Can you work these out from the model? Positions are in its coordinate system, mm. A direction names the side the tool comes from. Give positions to 0.01 mm unless a question says otherwise; leave off trailing zeros. Loops run counter-clockwise (first coordinate to the right, second up) from the corner with the lowest first, then second, coordinate; pieces in that order, holes last. Notation, with made-up numbers: M 66.5,1.25 L 122.5,1.25 A15 cw 122.5,29.25 Z; hole C -20.75,56 d5. An arc over 180 degrees is marked long. Put each result on its own line as item: value. Start each with the question number.
1) Imagine slicing it at B-B (z = -87.5). Write out the boundary of the cut face in (x, y).
2) For faces 1 (the cylindrical face through (2.535, 85.09, 84.615)), 2 (the flat face through (3, 0, -85)), which set-ups out of +Z, -Z, +X, -X, +Y, -Y let a thin tool reach every point of the face, with its end or its side?
3) If we mould it in two halves opening along Y, with no side actions, what happens to faces 3 (the flat face through (3, 10, 0)), 4 (the flat face through (2, 100, 1)), 5 (the flat face through (0, 1, 1))? For each: +Y half, -Y half, draft (parallel to the pull), parting line (faces both ways), or undercut.
4) Imagine slicing it at D-D (x = 1.5). State how many separate pieces and enclosed holes the cut face has, then the cut area to 3 significant figures.
5) Imagine slicing it at C-C (y = 74). Write out the boundary of the cut face in (x, z).
6) Please list where these lines run through material, in increasing order: line 1 along Z through (x, y) = (2.3, 6.5); line 2 along Y through (x, z) = (1.5, -50.5); line 3 along Y through (x, z) = (0.25, -21). Write a range as from..to.
7) Imagine slicing it at A-A (y = -38). Write out the boundary of the cut face in (x, z).
from build123d import *

# Parameters (mm, degrees)
SKETCH_1_W          = 200
SKETCH_1_H          = 200
SKETCH_1_R          = 5
EXTRUDE_1_DEPTH     = 5
SKETCH_3_R          = 2.1
CUT_EXTRUDE_2_DEPTH = 142.509716981


with BuildPart() as part:
    # 草图1 → 凸台-拉伸1 (new body)
    with BuildSketch(Plane(origin=(0, 0, 0), x_dir=(0, 0, -1), z_dir=(1, 0, 0))):
        Rectangle(SKETCH_1_W, SKETCH_1_H)
        with Locations((-50, 87.5)):
            Circle(SKETCH_1_R, mode=Mode.SUBTRACT)
        with Locations((50, 87.5)):
            Circle(SKETCH_1_R, mode=Mode.SUBTRACT)
        with Locations((-87.5, 50)):
            Circle(SKETCH_1_R, mode=Mode.SUBTRACT)
        with Locations((-87.5, -50)):
            Circle(SKETCH_1_R, mode=Mode.SUBTRACT)
        with Locations(Location((87.5, -50, 0), (0, 0, 180))):
            Circle(SKETCH_1_R, mode=Mode.SUBTRACT)
        with Locations(Location((87.5, 50, 0), (0, 0, 180))):
            Circle(SKETCH_1_R, mode=Mode.SUBTRACT)
    extrude(amount=EXTRUDE_1_DEPTH)

    # 草图3 → 切除-拉伸2 (cut, through all)
    with BuildSketch(Plane(origin=(5, 0, 0), x_dir=(0, 0, -1), z_dir=(1, 0, 0))):
        with Locations((-55, 20)):
            Circle(SKETCH_3_R)
        with Locations((-55, 0)):
            Circle(SKETCH_3_R)
        with Locations((-55, -20)):
            Circle(SKETCH_3_R)
        with Locations((55, 0)):
            Circle(SKETCH_3_R)
        with Locations((55, 20)):
            Circle(SKETCH_3_R)
        with Locations((55, -20)):
            Circle(SKETCH_3_R)
        with Locations((-35, 0)):
            Circle(SKETCH_3_R)
        with Locations((-15, 0)):
            Circle(SKETCH_3_R)
        with Locations((35, 0)):
            Circle(SKETCH_3_R)
        with Locations((15, 0)):
            Circle(SKETCH_3_R)
        with BuildLine():
            Line((-45, 66.143782777), (-45, 42.143782777))
            ThreePointArc((-45, 42.143782777), (0, 61.653048803), (45, 42.143782777))
            Line((45, 42.143782777), (45, 66.143782777))
            ThreePointArc((45, 66.143782777), (0, 80), (-45, 66.143782777))
        make_face()
        with BuildLine():
            Line((-45, -66.143782777), (-45, -42.143782777))
            ThreePointArc((-45, -42.143782777), (0, -61.653048803), (45, -42.143782777))
            Line((45, -42.143782777), (45, -66.143782777))
            ThreePointArc((45, -66.143782777), (0, -80), (-45, -66.143782777))
        make_face()
        with BuildLine():
            Line((-100, -66.332495807), (-100, -100))
            Line((-100, -100), (-66.332495807, -100))
            ThreePointArc((-66.332495807, -100), (-84.852813742, -84.852813742), (-100, -66.332495807))
        make_face()
        with BuildLine():
            Line((66.332495807, -100), (100, -100))
            Line((100, -100), (100, -66.332495807))
            ThreePointArc((100, -66.332495807), (84.852813742, -84.852813742), (66.332495807, -100))
        make_face()
        with BuildLine():
            Line((66.332495807, 100), (100, 100))
            Line((100, 100), (100, 66.332495807))
            ThreePointArc((100, 66.332495807), (84.852813742, 84.852813742), (66.332495807, 100))
        make_face()
        with BuildLine():
            Line((-100, 66.332495807), (-100, 100))
            Line((-100, 100), (-66.332495807, 100))
            ThreePointArc((-66.332495807, 100), (-84.852813742, 84.852813742), (-100, 66.332495807))
        make_face()
        with BuildLine():
            Line((-65, 35), (-65, -35))
            ThreePointArc((-65, -35), (-75, -45), (-85, -35))
            Line((-85, -35), (-85, 35))
            ThreePointArc((-85, 35), (-75, 45), (-65, 35))
        make_face()
        with BuildLine():
            Line((65, 35), (65, -35))
            ThreePointArc((65, -35), (75, -45), (85, -35))
            Line((85, -35), (85, 35))
            ThreePointArc((85, 35), (75, 45), (65, 35))
        make_face()
        with BuildLine():
            Line((-30, 30), (30, 30))
            ThreePointArc((30, 30), (40, 20), (30, 10))
            Line((30, 10), (-30, 10))
            ThreePointArc((-30, 10), (-40, 20), (-30, 30))
        make_face()
        with BuildLine():
            Line((-30, -30), (30, -30))
            ThreePointArc((30, -30), (40, -20), (30, -10))
            Line((30, -10), (-30, -10))
            ThreePointArc((-30, -10), (-40, -20), (-30, -30))
        make_face()
    extrude(amount=-CUT_EXTRUDE_2_DEPTH, mode=Mode.SUBTRACT)


solid = part.part
Recorded:
1. outline: M 0,-82.12 L 5,-82.12 L 5,-55 L 0,-55 Z; M 0,-45 L 5,-45 L 5,45 L 0,45 Z; M 0,55 L 5,55 L 5,82.12 L 0,82.12 Z
2. face 1: +Z, +X, -X, +Y
2. face 2: +X, -X
3. face 3: undercut
3. face 4: +Y half
3. face 5: draft
4. separate pieces: 1
4. enclosed holes: 22
4. area: 27,400 mm²
5. outline: M 0,-94.47 L 5,-94.47 L 5,-30.4 L 0,-30.4 Z; M 0,30.4 L 5,30.4 L 5,94.47 L 0,94.47 Z
6. line 1: -100..-85, -65..65, 85..100
6. line 2: -100..82.53, 92.47..100
6. line 3: -100..-77.19, -57.97..-30, -10..10, 30..57.97, 77.19..100
7. outline: M 0,-100 L 5,-100 L 5,-84.54 L 0,-84.54 Z; M 0,-65.46 L 5,-65.46 L 5,65.46 L 0,65.46 Z; M 0,84.54 L 5,84.54 L 5,100 L 0,100 Z
